```python
from build123d import *

# Parameters (mm, degrees)
F0_R     = 5
F1_DEPTH = 97
F2_DEPTH = 35
F3_R     = 5
F4_DEPTH = 58
F5_W     = 21.1601814699
F5_H     = 15
F5_W_2   = 38.8398185301
F6_DEPTH = 94.4868054059
F7_W     = 48.4832398096
F7_H     = 22
F7_W_2   = 11.5167601904
F8_DEPTH = 53.4786196206


with BuildPart() as f1:
    # F0 (on Front) → F1 (new body)
    with BuildSketch(Plane.XZ):
        with BuildLine():
            Line((-33.3940822773, -3.829139489), (-78.1385323231, -23.6095790069))
            ThreePointArc((-78.1385323231, -23.6095790069), (-83.2413837038, -36.7990030954), (-70.0519596153, -41.9018544761))
            Line((-70.0519596153, -41.9018544761), (-33.6129821019, -25.7930635521))
            ThreePointArc((-33.6129821019, -25.7930635521), (-16.8207912618, -34.9776541604), (0, -25.8455482049))
            ThreePointArc((0, -25.8455482049), (1.7560740266, -7.4903982751), (-12.2514262399, 4.5006509372))
            ThreePointArc((-12.2514262399, 4.5006509372), (-24.1207121326, 3.6302295915), (-33.3940822773, -3.829139489))
        make_face()
        with Locations((-74.0952459692, -32.7557167415)):
            Circle(F0_R, mode=Mode.SUBTRACT)
        with Locations((-16.789562501, -14.9776785413)):
            Circle(F0_R, mode=Mode.SUBTRACT)
    extrude(amount=F1_DEPTH)

    # F0 (on Front) → F2 (join)
    with BuildSketch(Plane.XZ):
        with BuildLine():
            Line((-33.3940822773, -3.829139489), (-78.1385323231, -23.6095790069))
            ThreePointArc((-78.1385323231, -23.6095790069), (-83.2413837038, -36.7990030954), (-70.0519596153, -41.9018544761))
            Line((-70.0519596153, -41.9018544761), (-33.6129821019, -25.7930635521))
            ThreePointArc((-33.6129821019, -25.7930635521), (-16.8207912618, -34.9776541604), (0, -25.8455482049))
            ThreePointArc((0, -25.8455482049), (1.7560740266, -7.4903982751), (-12.2514262399, 4.5006509372))
            ThreePointArc((-12.2514262399, 4.5006509372), (-24.1207121326, 3.6302295915), (-33.3940822773, -3.829139489))
        make_face()
        with Locations((-74.0952459692, -32.7557167415)):
            Circle(F0_R, mode=Mode.SUBTRACT)
        with Locations((-16.789562501, -14.9776785413)):
            Circle(F0_R, mode=Mode.SUBTRACT)
        with BuildLine():
            Line((101.7329280454, 10.2593952934), (-12.2514262399, 4.5006509372))
            ThreePointArc((-12.2514262399, 4.5006509372), (1.7560740266, -7.4903982751), (0, -25.8455482049))
            Line((0, -25.8455482049), (103.7832955951, -9.6076711141))
            ThreePointArc((103.7832955951, -9.6076711141), (92.2903408389, -0.7544573444), (101.7329280454, 10.2593952934))
        make_face()
        with BuildLine():
            ThreePointArc((112.2375068401, 0.2721333944), (109.1278701125, 7.5194014295), (101.7329280454, 10.2593952934))
            ThreePointArc((101.7329280454, 10.2593952934), (92.2903408389, -0.7544573444), (103.7832955951, -9.6076711141))
            ThreePointArc((103.7832955951, -9.6076711141), (109.8354633926, -6.2294861135), (112.2375068401, 0.2721333944))
        make_face()
        with Locations((102.2375068401, 0.2721333944)):
            Circle(F0_R, mode=Mode.SUBTRACT)
    extrude(amount=F2_DEPTH)

    # F3 (on face) → F4 (cut)
    with BuildSketch(Plane(origin=(0, 0, 0), x_dir=(-1, 0, 0), z_dir=(0, 1, 0))):
        with BuildLine():
            ThreePointArc((33.3940822773, -3.829139489), (31.8014961432, -14.0586725369), (25.3075095695, -22.1214149583))
            Line((25.3075095695, -22.1214149583), (33.6129821019, -25.7930635521))
            Line((33.6129821019, -25.7930635521), (70.0519596153, -41.9018544761))
            ThreePointArc((70.0519596153, -41.9018544761), (64.9491082346, -28.7124303876), (78.1385323231, -23.6095790069))
            Line((78.1385323231, -23.6095790069), (33.3940822773, -3.829139489))
        make_face()
        with BuildLine():
            ThreePointArc((84.0952459692, -32.7557167415), (82.4747705243, -27.2982843571), (78.1385323231, -23.6095790069))
            ThreePointArc((78.1385323231, -23.6095790069), (64.9491082346, -28.7124303876), (70.0519596153, -41.9018544761))
            ThreePointArc((70.0519596153, -41.9018544761), (79.5526783536, -41.1352412966), (84.0952459692, -32.7557167415))
        make_face()
        with Locations((74.0952459692, -32.7557167415)):
            Circle(F3_R, mode=Mode.SUBTRACT)
    extrude(amount=-F4_DEPTH, mode=Mode.SUBTRACT)

    # F5 (on face) → F6 (cut, through all)
    with BuildSketch(Plane(origin=(-4.0432863539, 0, 9.1461377346), x_dir=(0.9146137735, 0, 0.4043286354), z_dir=(-0.4043286354, 0, 0.9146137735))):
        with Locations((-91.5926974976, -77.5)):
            Rectangle(F5_W, F5_H)
        with Locations((-61.5926974976, -77.5)):
            Rectangle(F5_W_2, F5_H)
    extrude(amount=-F6_DEPTH, mode=Mode.SUBTRACT)

    # F7 (on face) → F8 (cut, through all)
    with BuildSketch(Plane(origin=(-0.2579961306, 0, 5.1065858341), x_dir=(0.9987261899, 0, 0.0504578795), z_dir=(-0.0504578795, 0, 0.9987261899))):
        with Locations((77.8793870409, -19)):
            Rectangle(F7_W, F7_H)
        with Locations((107.8793870409, -19)):
            Rectangle(F7_W_2, F7_H)
    extrude(amount=-F8_DEPTH, mode=Mode.SUBTRACT)


solid = f1.part
```
Model file for the job. Use its own axes, mm. A direction names the side the tool comes from. Coordinates: 2 decimals unless noted, no trailing zeros. Order: outer loops, then holes, each group sorted by start corner. A loop starts at its lowest first (then second) coordinate and runs counter-clockwise, first axis right, second up. Notation, with made-up numbers: (87.5, -7.5) -> (124.5, -7.5) arc R21 ccw to (124.5, 4.5) -> close; hole circle Ø10 at (1, -15.5). An arc over 180 degrees is marked (long way). Answer as a JSON object with one key per item and string values. Group by question number.
1) Cut at D-D, the plane x = -50.5. Write the cut outline in (y, z).
2) Flat gauge pins, fed straight in: pin 1 (10 mm diameter, centred on x = -19.5, y = -21, fed in from -Z); pin 2 (4 mm diameter, centred on x = -9.5, y = -65, fed in from -Z); pin 3 (2 mm diameter, centred on y = -24, z = -3, fed in from +X). Where does each tip first touch, or does it go through?
3) Cut at A-A, the plane x = 85. Write the cut outline in (y, z).
4) Cut at B-B, the plane y = -24. Write the cut outline in (x, z).
5) Which spindle directions (+Z, -Z, +X, -X, +Y, -Y) get a long thin tool onto all of the face, cutting with end or side? Do faces 1 (the face through (32.87, -17.26, 6.78)), 2 (the face through (97.242, -3.944, 0.492)), 3 (the face through (53.937, -19.154, -4.571)), 4 (the face through (-52.09, -85.89, -33.96)), 5 (the face through (22, 0, -7)). Say none if no direction does.
6) Pull direction X, two halves, no side cores. Call faces 6 (the face through (97.242, -32.465, 0.492)), 7 (the face through (-29.4, -28.59, -23.93)), 8 (the face through (-83.328, -63.916, -36.597)): +X half, -X half, draft (parallel to the pull), parting line (faces both ways), or undercut.
7) Cut at C-C, the plane y = -89.5. Write the cut outline in (x, z).
8) Drill centre lines: L1, parallel to Y at x = 39.5, z = -17; L2, parallel to Y at x = 67, z = -1; L3, parallel to Z at x = -75, y = -67. Where is each one in solid material? Low to high.
Check values:
{
 "1": {"outline": "(-97, -33.26) -> (-85, -33.26) -> (-85, -11.39) -> (-97, -11.39) -> close; (-70, -33.26) -> (-58, -33.26) -> (-58, -11.39) -> (-70, -11.39) -> close"},
 "2": {"pin 1": "stops at z = -34.98", "pin 2": "stops at z = -34.27", "pin 3": "stops at x = 53.91"},
 "3": {"outline": "(-35, -12.55) -> (-30, -12.55) -> (-30, 9.41) -> (-35, 9.41) -> close; (-8, -12.55) -> (0, -12.55) -> (0, 9.41) -> (-8, 9.41) -> close"},
 "4": {"outline": "(-33.61, -25.79) arc R20 ccw to (0, -25.85) -> (54.58, -17.31) -> (53.31, 7.81) -> (-12.25, 4.5) arc R20 ccw to (-33.39, -3.83) arc R20 ccw to (-25.31, -22.12) -> close; hole circle Ø10 at (-16.79, -14.98)"},
 "5": {"face 1": "+Z, +Y, -Y", "face 2": "+Y, -Y", "face 3": "+Z, +X", "face 4": "-Z, +Y, -Y", "face 5": "+Z, -Z, +X, -X, +Y"},
 "6": {"face 6": "undercut", "face 7": "-X half", "face 8": "parting line"},
 "7": {"outline": "(-78.14, -23.61) arc R10 ccw to (-70.05, -41.9) -> (-33.61, -25.79) arc R20 ccw (long way) to (-33.39, -3.83) -> close; hole circle Ø10 at (-74.1, -32.76); hole circle Ø10 at (-16.79, -14.98)"},
 "8": {"L1": "y = -35 to 0", "L2": "y = -35 to -30, -8 to 0", "L3": "z = -42.71 to -37.67, -27.84 to -22.22"}
}
